The model under review builds one solid part; all positions refer to its coordinate system, in mm. A direction names the side the tool comes from. Coordinates: 2 decimals unless noted, no trailing zeros. Write each loop counter-clockwise with the first axis right and the second up, starting at its lowest first coordinate (ties: lowest second). Pieces come first, ordered by that corner, then holes. Notation, with made-up numbers: M -14.5,60 L 31.5,60 A20 cw 31.5,74 Z; hole C 32.25,54.25 d1. An arc over 180 degrees is marked long. Answer as a JSON object with one key per item and string values.
```python
from build123d import *

# Parameters (mm, degrees)
SKETCH1_W           = 25.4
SKETCH1_H           = 25.4
SKETCH1_W_2         = 22.225
SKETCH1_H_2         = 22.225
BOSS_EXTRUDE1_DEPTH = 50.8
SKETCH2_R           = 12.7
CUT_EXTRUDE1_DEPTH  = 54.881536726
SKETCH3_R           = 3.175
CUT_EXTRUDE2_DEPTH  = 59.198711326


with BuildPart() as part:
    # Sketch1 → Boss-Extrude1 (new body)
    with BuildSketch(Plane(origin=(0, 0, 0), x_dir=(1, 0, 0), z_dir=(0, 1, 0))):
        Rectangle(SKETCH1_W, SKETCH1_H)
        Rectangle(SKETCH1_W_2, SKETCH1_H_2, mode=Mode.SUBTRACT)
    extrude(amount=BOSS_EXTRUDE1_DEPTH)

    # Sketch2 → Cut-Extrude1 (cut, through all)
    with BuildSketch(Plane(origin=(0, 50.8, 0), x_dir=(1, 0, 0), z_dir=(0, 1, 0))):
        with Locations((12.7, 0)):
            Circle(SKETCH2_R)
    extrude(amount=-CUT_EXTRUDE1_DEPTH, mode=Mode.SUBTRACT)

    # Sketch3 → Cut-Extrude2 (cut, through all)
    with BuildSketch(Plane(origin=(0, 0, -12.7), x_dir=(-1, 0, 0), z_dir=(0, 0, -1))):
        with Locations((6.35, 44.45)):
            Circle(SKETCH3_R)
        with Locations((6.35, 6.35)):
            Circle(SKETCH3_R)
    extrude(amount=-CUT_EXTRUDE2_DEPTH, mode=Mode.SUBTRACT)


solid = part.part
```
(1) For faces 5 (the face through (-2, 25, -11.112)), 6 (the face through (-12.7, 25, 0)), list the 3-axis set-ups (+Z, -Z, +X, -X, +Y, -Y) from which the entire face can be reached by the end or side of a thin tool; tool diameter is ignored.
Results list:
{"face 5": "+X, +Y, -Y", "face 6": "+Z, -Z, -X, +Y, -Y"}
(2) Add section B-B on y = 6.35. Give the boundary of the cut face in (x, z) (1 decimal), and give its area (3 significant figures).
Results list:
{"outline": "M -12.7,-12.7 L -9.5,-12.7 L -9.5,-11.1 L -11.1,-11.1 L -11.1,11.1 L -9.5,11.1 L -9.5,12.7 L -12.7,12.7 Z; M -3.2,-12.7 L 12.7,-12.7 A12.7 cw 6.6,-11.1 L -3.2,-11.1 Z; M -3.2,11.1 L 6.6,11.1 A12.7 cw 12.7,12.7 L -3.2,12.7 Z", "area": "82.6 mm²"}
(3) Draft analysis for pull direction Z (two halves, no side actions). For faces 1 (the face through (-11.3, 50.8, -0.1)), 2 (the face through (0, 25, 12.7)), 3 (the face through (-11.112, 25, 0)), 4 (the face through (0, 25, -12.7)), state which applies: released by +Z, released by -Z, zero draft, split by the parting line, or undercut.
Results list:
{"face 1": "zero draft", "face 2": "released by +Z", "face 3": "undercut", "face 4": "released by -Z"}
(4) Add section D-D on y = 14.5. Give the boundary of the cut face in (x, z), and give its area (3 significant figures).
Results list:
{"outline": "M -12.7,-12.7 L 12.7,-12.7 A12.7 cw 6.55,-11.11 L -11.11,-11.11 L -11.11,11.11 L 6.55,11.11 A12.7 cw 12.7,12.7 L -12.7,12.7 Z", "area": "103 mm²"}
(5) Add section A-A on x = -1.25. Give the boundary of the cut face in (y, z), and give its area (3 significant figures).
Results list:
{"outline": "M 0,-12.7 L 50.8,-12.7 L 50.8,-11.11 L 0,-11.11 Z; M 0,11.11 L 50.8,11.11 L 50.8,12.7 L 0,12.7 Z", "area": "161 mm²"}
(6) Wall thickness on line 1 along Y through (x, z) = (-6.35, -11.9) (3 decimals); line 2 along Z through (x, y) = (2.25, 24); line 3 along X through (y, z) = (25, -9.25): over which ranges is each line inside the solid? List them lowest first. Write a range as from..to.
Results list:
{"line 1": "0..3.175, 9.525..41.275, 47.625..50.8", "line 2": "-12.7..-11.11, 11.11..12.7", "line 3": "-12.7..-11.11"}
(7) For pin 1 Ø5.5 at (x, y) = (-6.35, 6.35) entering from +Z, flat-tipped, find the tip position at first contact; note if it passes through.
Results list:
{"pin 1": "through"}
(8) Add section C-C on x = -6.35. Give the boundary of the cut face in (y, z) (1 decimal), and give its area (3 significant figures).
Results list:
{"outline": "M 0,-12.7 L 3.2,-12.7 L 3.2,-11.1 L 0,-11.1 Z; M 0,11.1 L 3.2,11.1 L 3.2,12.7 L 0,12.7 Z; M 9.5,-12.7 L 41.3,-12.7 L 41.3,-11.1 L 9.5,-11.1 Z; M 9.5,11.1 L 41.3,11.1 L 41.3,12.7 L 9.5,12.7 Z; M 47.6,-12.7 L 50.8,-12.7 L 50.8,-11.1 L 47.6,-11.1 Z; M 47.6,11.1 L 50.8,11.1 L 50.8,12.7 L 47.6,12.7 Z", "area": "121 mm²"}
